Autodesk Inventor part; units mm, degrees
ref_plane "C1_XY" through (0, 0, 0) normal (0, 0, 1) x (1, 0, 0)
ref_plane "C1_YZ" through (0, 0, 0) normal (1, 0, 0) x (0, 1, 0)
ref_plane "C1_ZX" through (0, 0, 0) normal (0, 1, 0) x (0, 0, 1)
sketch "Sketch_1" plane through (0, 0, 0) normal (0, 0, 1) x (1, 0, 0)
  line L0 (-15, -4) -> (-15, -13)
  arc A0 (-15, -13) -> (-13, -15) centre (-13, -13) ccw
  line L1 (-13, -15) -> (-4, -15)
  line L2 (-4, -15) -> (-4, -13)
  line L3 (-4, -13) -> (-8.25, -13)
  line L4 (-8.25, -13) -> (-8.25, -9.6642)
  line L5 (-8.25, -9.6642) -> (-4.5858, -6)
  line L6 (-4.5858, -6) -> (-0.5196, -6)
  line L7 (-0.5196, -6) -> (0, -5.7)
  line L8 (0, -5.7) -> (0.5196, -6)
  line L9 (0.5196, -6) -> (4.5858, -6)
  line L10 (4.5858, -6) -> (8.25, -9.6642)
  line L11 (8.25, -9.6642) -> (8.25, -13)
  line L12 (8.25, -13) -> (4, -13)
  line L13 (4, -13) -> (4, -15)
  line L14 (4, -15) -> (13, -15)
  arc A1 (13, -15) -> (15, -13) centre (13, -13) ccw
  line L15 (15, -13) -> (15, -4)
  line L16 (15, -4) -> (13, -4)
  line L17 (13, -4) -> (13, -8.25)
  line L18 (13, -8.25) -> (9.6642, -8.25)
  line L19 (9.6642, -8.25) -> (6, -4.5858)
  line L20 (6, -4.5858) -> (6, -0.5196)
  line L21 (6, -0.5196) -> (5.7, 0)
  line L22 (5.7, 0) -> (6, 0.5196)
  line L23 (6, 0.5196) -> (6, 4.5858)
  line L24 (6, 4.5858) -> (9.6642, 8.25)
  line L25 (9.6642, 8.25) -> (13, 8.25)
  line L26 (13, 8.25) -> (13, 4)
  line L27 (13, 4) -> (15, 4)
  line L28 (15, 4) -> (15, 13)
  arc A2 (15, 13) -> (13, 15) centre (13, 13) ccw
  line L29 (13, 15) -> (4, 15)
  line L30 (4, 15) -> (4, 13)
  line L31 (4, 13) -> (8.25, 13)
  line L32 (8.25, 13) -> (8.25, 9.6642)
  line L33 (8.25, 9.6642) -> (4.5858, 6)
  line L34 (4.5858, 6) -> (0.5196, 6)
  line L35 (0.5196, 6) -> (0, 5.7)
  line L36 (0, 5.7) -> (-0.5196, 6)
  line L37 (-0.5196, 6) -> (-4.5858, 6)
  line L38 (-4.5858, 6) -> (-8.25, 9.6642)
  line L39 (-8.25, 9.6642) -> (-8.25, 13)
  line L40 (-8.25, 13) -> (-4, 13)
  line L41 (-4, 13) -> (-4, 15)
  line L42 (-4, 15) -> (-13, 15)
  arc A3 (-13, 15) -> (-15, 13) centre (-13, 13) ccw
  line L43 (-15, 13) -> (-15, 4)
  line L44 (-15, 4) -> (-13, 4)
  line L45 (-13, 4) -> (-13, 8.25)
  line L46 (-13, 8.25) -> (-9.6642, 8.25)
  line L47 (-9.6642, 8.25) -> (-6, 4.5858)
  line L48 (-6, 4.5858) -> (-6, 0.5196)
  line L49 (-6, 0.5196) -> (-5.7, 0)
  line L50 (-5.7, 0) -> (-6, -0.5196)
  line L51 (-6, -0.5196) -> (-6, -4.5858)
  line L52 (-6, -4.5858) -> (-9.6642, -8.25)
  line L53 (-9.6642, -8.25) -> (-13, -8.25)
  line L54 (-13, -8.25) -> (-13, -4)
  line L55 (-13, -4) -> (-15, -4)
extrude "Extrusion1" add sketch "Sketch_1" against normal blind 690
sketch "Sketch2" plane through (0, 0, -690) normal (0, 0, -1) x (-1, 0, 0)
  point P0 (0, 0)
hole "Hole1" at (0, 0, -690) direction (0, 0, 1) diameter 6.8 depth 690
sketch "Sketch3" plane through (0, 0, -690) normal (0, 0, -1) x (-1, 0, 0)
  point P0 (-11.6, 11.6)
hole "Hole2" at (11.6, 11.6, -690) direction (0, 0, 1) diameter 4.2 depth 690
pattern_linear "Rectangular Pattern1" count 2 spacing 23.2 along (-1, 0, 0) count 2 spacing 23.2 along (0, -1, 0) of "Hole2"
ref_plane "C1_XY" through (0, 0, 0) normal (0, 0, 1) x (1, 0, 0)
ref_plane "C1_YZ" through (0, 0, 0) normal (1, 0, 0) x (0, 1, 0)
ref_plane "C1_ZX" through (0, 0, 0) normal (0, 1, 0) x (0, 0, 1)
ref_plane "to_frame_cap1_XY" through (0, 0, 0) normal (0, 0, 1) x (1, 0, 0)
ref_plane "to_frame_cap1_YZ" through (0, 0, 0) normal (1, 0, 0) x (0, 1, 0)
ref_plane "to_frame_cap1_ZX" through (0, 0, 0) normal (0, 1, 0) x (0, 0, 1)
ref_plane "to_frame_cap2_XY" through (0, 0, -690) normal (0, 0, -1) x (1, 0, 0)
ref_plane "to_frame_cap2_YZ" through (0, 0, -690) normal (1, 0, 0) x (0, -1, 0)
ref_plane "to_frame_cap2_ZX" through (0, 0, -690) normal (0, -1, 0) x (0, 0, -1)
properties part number "HFS6-3030-690"
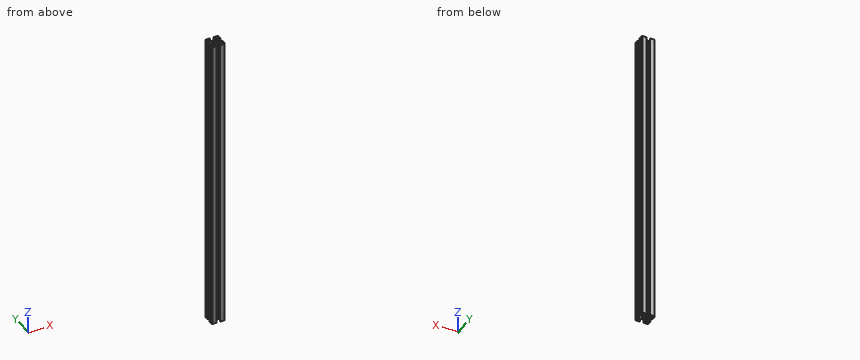
Geometry check sheet. Reference: the model listing, model coordinates, mm. Round coordinates to 2 decimals unless told otherwise and drop trailing zeros. Put each result on its own line as item: value.
1) Thickness scan on probe 1 along Y at (x, z) = (-11.6, -451); probe 2 along X at (y, z) = (11, -264). Record the ranges inside material, lowest first. Write a range as from..to.
Recorded:
probe 1: y = -15..-13.7, -9.5..-8.25, 8.25..9.5, 13.7..15
probe 2: x = -15..-13.61, -9.59..-8.25, 8.25..9.59, 13.61..15
2) Depth check by flat-ended pin: P1, Ø1, axis at y = -3, z = -472.5, coming from the +X side; P2, Ø2, axis at y = 14.5, z = -463, coming from the -X side; P3, Ø4, axis at x = 5, y = -10, coming from the +Z side; P4, Ø1, axis at x = 14, z = -236, coming from the +Y side. Enter the tip coordinate at first touch or a pass-through.
Recorded:
P1: stops at x = 6
P2: stops at x = -14.94
P3: passes through
P4: stops at y = 14.94
3) Cross-section at A-A, the plane z = -535. Give the number of separate pieces and of enclosed holes in the cut face, plus the area to 3 significant figures.
Recorded:
separate pieces: 1
enclosed holes: 5
area: 332 mm2
